Can you work these out from the model? Positions are in its coordinate system, mm. Face numbers are marked on the shaded views. A direction names the side the tool comes from. Give positions to 0.01 mm unless a question says otherwise; leave off trailing zeros. Write each loop counter-clockwise with the first axis right and the second up, starting at its lowest first coordinate (ties: lowest second). Pieces come first, ordered by that corner, then holes. Notation, with made-up numbers: (-30.75, 59.5) -> (-26.75, 59.5) arc R23 cw to (-26.75, 71.5) -> close; hole circle Ø7 at (35, 19.25). An arc over 180 degrees is marked (long way). One line per item, written item: value.
from build123d import *
from OCP.BRepFilletAPI import BRepFilletAPI_MakeFillet

# Parameters (mm, degrees)
CROQUIS1_R              = 5.375
SALIENTE_EXTRUIR1_DEPTH = 6
CROQUIS2_R              = 6.5
SALIENTE_EXTRUIR2_DEPTH = 2
VACIADO1_T              = -1
SALIENTE_EXTRUIR3_START = 4.5
CROQUIS3_R              = 4.375
SALIENTE_EXTRUIR3_DEPTH = 4.5
REDONDEO1_R1            = 0.5
REDONDEO1_R2            = 1


with BuildPart() as part:
    # Croquis1 → Saliente-Extruir1 (new body)
    with BuildSketch(Plane(origin=(0, 0, 0), x_dir=(1, 0, 0), z_dir=(0, 1, 0))):
        with Locations(Location((0, 0, 0), (0, 0, 270))):
            Circle(CROQUIS1_R)
    extrude(amount=SALIENTE_EXTRUIR1_DEPTH)

    # Croquis2 → Saliente-Extruir2 (add)
    with BuildSketch(Plane.XZ):
        with Locations(Location((0, 0, 0), (0, 0, 270))):
            Circle(CROQUIS2_R)
    extrude(amount=SALIENTE_EXTRUIR2_DEPTH)

    # Vaciado1
    vaciado1_openings = [part.faces().sort_by_distance(p)[0] for p in [
        (0, -2, 0),
    ]]
    offset(amount=VACIADO1_T, openings=vaciado1_openings, kind=Kind.INTERSECTION)

    # Croquis3 → Saliente-Extruir3 (add)
    with BuildSketch(Plane.XZ.offset(-5).offset(SALIENTE_EXTRUIR3_START)):
        with Locations(Location((0, 0, 0), (0, 0, 270))):
            Circle(CROQUIS3_R)
    extrude(amount=-SALIENTE_EXTRUIR3_DEPTH)

    # Redondeo1: one fillet with a radius per group of edges: ONE call of the kernel's fillet builder (fillet() takes one radius for all edges)
    redondeo1_edges_1 = [part.edges().sort_by_distance(p)[0] for p in [
        (0, 6, -5.375),
    ]]
    redondeo1_edges_2 = [part.edges().sort_by_distance(p)[0] for p in [
        (0, 0, 6.5),
    ]]
    redondeo1 = BRepFilletAPI_MakeFillet(part.part.solid().wrapped)
    for e in redondeo1_edges_1:
        redondeo1.Add(REDONDEO1_R1, e.wrapped)
    for e in redondeo1_edges_2:
        redondeo1.Add(REDONDEO1_R2, e.wrapped)
    add(Compound.cast(redondeo1.Shape()), mode=Mode.REPLACE)

    # Croquis4 → Cortar-Revoluci_n4 (revolve, cut)
    with BuildSketch(Plane.XY):
        with BuildLine():
            Line((0, 20), (0, 5.175505911))
            ThreePointArc((0, 5.175505911), (-14.824494089, 20), (0, 34.824494089))
            Line((0, 34.824494089), (0, 20))
        make_face()
    revolve(axis=Axis((0, 20, 0), (0, -1, 0)), mode=Mode.SUBTRACT)


solid = part.part
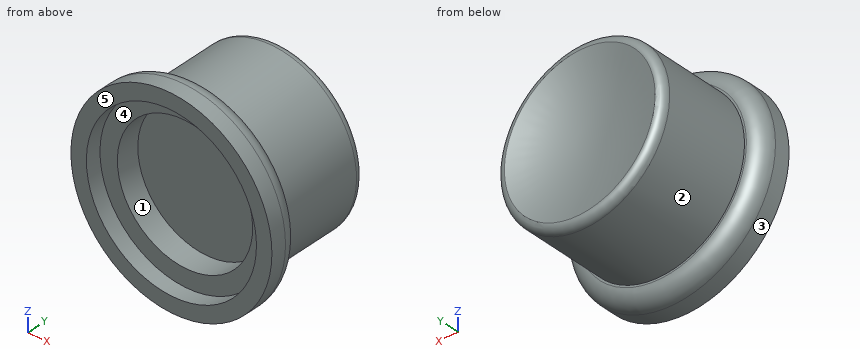
1) I need wall thicknesses on L1, parallel to X at y = -1.35, z = 0; L2, parallel to X at y = -0.2, z = 0 (3 decimals); L3, parallel to Y at x = 5, z = 0. Which ranges of each line are inside material? Lowest first, please.
Answer list:
L1: x = -6.5 to -5.5, 5.5 to 6.5
L2: x = -6.1 to -4.375, 4.375 to 6.1
L3: y = -1 to 5.98
2) We'd pull the mould along Z, two halves only. Please class the marked faces 3, 4 and 5: released by +Z, released by -Z, zero draft, split by the parting line, or undercut.
Answer list:
face 3: split by the parting line
face 4: undercut
face 5: zero draft
3) For the marked faces 1 and 2, which set-ups out of +Z, -Z, +X, -X, +Y, -Y let a thin tool reach every point of the face, with its end or its side?
Answer list:
face 1: -Y
face 2: +Y
4) If we section it at C-C (y = 2.5): Write out the boundary of the cut face in (x, z) (3 decimals), and give its area (3 significant figures).
Answer list:
outline: circle Ø10.75 at (0, 0)
area: 90.8 mm^2
5) Will these pins go through, and if not, where does the flat tip stop? pin 1 (1.5 mm diameter, centred on y = 0, z = 0, fed in from -X); pin 2 (4.5 mm diameter, centred on x = 0, z = 0, fed in from -Y); pin 3 (1.5 mm diameter, centred on x = -5, z = -4, fed in from +Y).
Answer list:
pin 1: stops at x = -6.47
pin 2: stops at y = 0.5
pin 3: stops at y = -0.01
